Autodesk Inventor part; units mm, degrees
ref_plane "YZ Plane" through (0, 0, 0) normal (1, 0, 0) x (0, 1, 0)
ref_plane "XZ Plane" through (0, 0, 0) normal (0, 1, 0) x (-1, 0, 0)
ref_plane "XY Plane" through (0, 0, 0) normal (0, 0, 1) x (1, 0, 0)
sketch "Sketch1" plane through (0, 0, 0) normal (0, 1, 0) x (-1, 0, 0)
  line L0 (-26, 36) -> (26, 36)
  line L1 (26, 36) -> (26, -36)
  line L2 (26, -36) -> (-26, -36)
  line L3 (-26, -36) -> (-26, 36)
  line L4 (-26, 36) -> (26, -36) construction
  line L5 (26, 36) -> (-26, -36) construction
  point P0 (0, 0)
  dimension "d0" = 72
  dimension "d1" = 52
extrude "Extrusion1" add sketch "Sketch1" along normal blind 1.6
sketch "Sketch2" plane through (0, 1.6, 0) normal (0, 1, 0) x (1, 0, 0)
  line L0 (-12.5, -33) -> (23, -33) construction
  line L1 (23, -33) -> (23, 33) construction
  line L2 (23, 33) -> (-12.5, 33) construction
  line L3 (-12.5, 33) -> (-12.5, -33) construction
  line L4 (-12.5, -33) -> (23, 33) construction
  line L5 (23, -33) -> (-12.5, 33) construction
  line L6 (26, 36) -> (-26, 36) construction
  line L7 (-26, -36) -> (26, -36) construction
  line L8 (26, -36) -> (26, 36) construction
  line L9 (26, 36) -> (-26, 36) construction
  line L10 (-26, 36) -> (-26, -36) construction
  point P0 (0, 0)
  point P1 (5.25, 0)
  dimension "d4" = 66
  dimension "d5" = 35.5
  dimension "d6" = 3
  dimension "d7" = 3
hole "Hole1" at (-12.5, 1.6, 33) at (-12.5, 1.6, -33) at (23, 1.6, -33) at (23, 1.6, 33) direction (0, -1, 0) diameter 3 end through all
sketch "Sketch3" plane through (0, 1.6, 0) normal (0, 1, 0) x (1, 0, 0)
  line L0 (13, -9) -> (25, -9)
  line L1 (25, -9) -> (25, 29)
  line L2 (25, 29) -> (13, 29)
  line L3 (13, 29) -> (13, -9)
  circle A0 centre (23, 33) radius 1.5 construction
  line L4 (26, -36) -> (26, 36) construction
  point P0 (0, 0)
  dimension "d15" = 38
  dimension "d16" = 12
  dimension "d18" = 4
  dimension "d19" = 1
extrude "Extrusion2" add sketch "Sketch3" along normal blind 14
sketch "Sketch4" plane through (0, 1.6, 0) normal (0, 1, 0) x (1, 0, 0)
  line L0 (7, -33) -> (23, -33)
  line L1 (23, -33) -> (23, -11)
  line L2 (23, -11) -> (7, -11)
  line L3 (7, -11) -> (7, -33)
  line L4 (13, -9) -> (13, 29) construction
  line L5 (13, 29) -> (25, 29) construction
  line L6 (25, 29) -> (25, -9) construction
  line L7 (25, -9) -> (13, -9) construction
  circle A0 centre (23, 33) radius 1.5 construction
  circle A1 centre (-12.5, -33) radius 1.5 construction
  circle A2 centre (-12.5, 33) radius 1.5 construction
  circle A3 centre (23, -33) radius 1.5 construction
  line L8 (-26, -36) -> (26, -36) construction
  line L9 (26, -36) -> (26, 36) construction
  line L10 (26, 36) -> (-26, 36) construction
  line L11 (-26, 36) -> (-26, -36) construction
  point P0 (0, 0)
  dimension "d22" = 22
  dimension "d23" = 16
extrude "Extrusion3" add sketch "Sketch4" along normal blind 15
sketch "Sketch5" plane through (0, 1.6, 0) normal (0, 1, 0) x (1, 0, 0)
  line L0 (-25, -28) -> (-6, -28)
  line L1 (-6, -28) -> (-6, 27)
  line L2 (-6, 27) -> (-25, 27)
  line L3 (-25, 27) -> (-25, -28)
  line L4 (-26, -36) -> (26, -36)
  line L5 (-26, 36) -> (-26, -36)
  point P0 (0, 0)
  dimension "d26" = 55
  dimension "d27" = 19
  dimension "d28" = 8
  dimension "d29" = 1
extrude "Extrusion4" add sketch "Sketch5" along normal blind 16
sketch "Sketch6" plane through (0, 0, 0) normal (0, -1, 0) x (1, 0, 0)
  circle A0 centre (23, 33) radius 1.5
  circle A1 centre (23, -33) radius 1.5
  circle A2 centre (-12.5, -33) radius 1.5
  circle A3 centre (-12.5, 33) radius 1.5
  line L0 (25.75, 31.4123) -> (23, 29.8246)
  line L1 (23, 29.8246) -> (20.25, 31.4123)
  line L2 (20.25, 31.4123) -> (20.25, 34.5877)
  line L3 (20.25, 34.5877) -> (23, 36.1754)
  line L4 (23, 36.1754) -> (25.75, 34.5877)
  line L5 (25.75, 34.5877) -> (25.75, 31.4123)
  line L6 (20.25, -31.4123) -> (23, -29.8246)
  line L7 (23, -29.8246) -> (25.75, -31.4123)
  line L8 (25.75, -31.4123) -> (25.75, -34.5877)
  line L9 (25.75, -34.5877) -> (23, -36.1754)
  line L10 (23, -36.1754) -> (20.25, -34.5877)
  line L11 (20.25, -34.5877) -> (20.25, -31.4123)
  line L12 (-9.75, 31.4123) -> (-12.5, 29.8246)
  line L13 (-12.5, 29.8246) -> (-15.25, 31.4123)
  line L14 (-15.25, 31.4123) -> (-15.25, 34.5877)
  line L15 (-15.25, 34.5877) -> (-12.5, 36.1754)
  line L16 (-12.5, 36.1754) -> (-9.75, 34.5877)
  line L17 (-9.75, 34.5877) -> (-9.75, 31.4123)
  line L18 (-9.75, -31.4123) -> (-9.75, -34.5877)
  line L19 (-9.75, -34.5877) -> (-12.5, -36.1754)
  line L20 (-12.5, -36.1754) -> (-15.25, -34.5877)
  line L21 (-15.25, -34.5877) -> (-15.25, -31.4123)
  line L22 (-15.25, -31.4123) -> (-12.5, -29.8246)
  line L23 (-12.5, -29.8246) -> (-9.75, -31.4123)
  line L24 (26, -36) -> (26, 36)
  line L25 (-26, 36) -> (-26, -36)
  point P0 (0, 0)
  dimension "d32" = 5.5
  dimension "d33" = 5.5
  dimension "d34" = 5.5
  dimension "d35" = 5.5
extrude "Extrusion5" add sketch "Sketch6" along normal blind 5
properties part number "backboard"
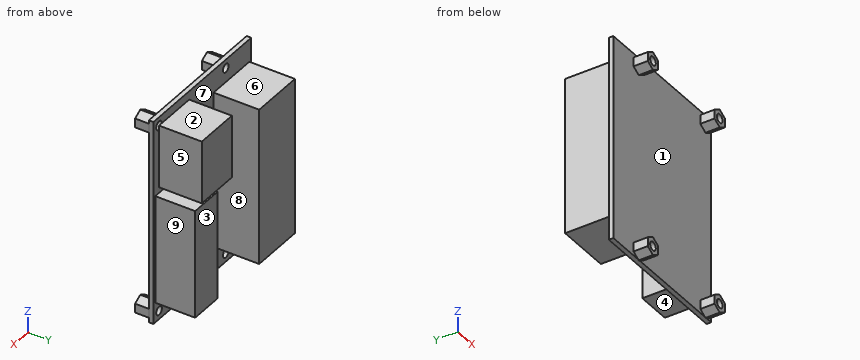
Work out the finished part from the listing and answer in its coordinate system (mm). Face numbers are marked on the shaded views. A direction names the side the tool comes from. Coordinates: 2 decimals unless noted, no trailing zeros. Write each loop counter-clockwise with the first axis right and the second up, starting at its lowest first coordinate (ties: lowest second). Pieces come first, ordered by that corner, then holes.
1. Flat-ended cylindrical pins translate along their axes: pin 1 (10 mm diameter, centred on x = -7, y = 1.5, fed in from -Z); pin 2 (3.5 mm diameter, centred on x = 22, y = 9.5, fed in from +Z); pin 3 (3 mm diameter, centred on x = -5.5, y = 7, fed in from +Z). Find the tip coordinate at first contact, or state that the pin passes through.
Results list:
pin 1: stops at z = -36
pin 2: stops at z = 33
pin 3: stops at z = 28
2. For the marked faces 1, 2, 3, 4 and 5, determine the directions among +Z, -Z, +X, -X, +Y, -Y from which every point of the face is accessible in a straight line to the end or side of a thin tool.
Results list:
face 1: -Y
face 2: +Z, +X, -X, +Y
face 3: -Z, +X, +Y
face 4: -Z, +X, -X, +Y
face 5: +Z, +X, +Y
3. The part is cut by section C-C, the plane x = -8. Write down the section's boundary in (y, z).
Results list:
outline: (0, -36) - (1.6, -36) - (1.6, -27) - (17.6, -27) - (17.6, 28) - (1.6, 28) - (1.6, 36) - (0, 36) - close
4. For a pull along X with two mould halves and no side action, classify the marked faces 6, 7, 8 and 9 as +X half, -X half, draft (parallel to the pull), parting line (faces both ways), or undercut.
Results list:
face 6: draft
face 7: undercut
face 8: undercut
face 9: +X half
5. The part is cut by section A-A, the plane y = 6. Write down the section's boundary in (x, z).
Results list:
outline: (-25, -27) - (-6, -27) - (-6, 28) - (-25, 28) - close; (7, 11) - (23, 11) - (23, 33) - (7, 33) - close; (13, -29) - (25, -29) - (25, 9) - (13, 9) - close
6. Consider line 1 along X through (y, z) = (-3.95, 33); line 2 along X through (y, z) = (0.45, -33); line 3 along Z through (x, y) = (-12.5, 0.3). Determine where each line is inside the solid, lowest interval first.
Results list:
line 1: x = -15.25 to -14, -11 to -9.75, 20.25 to 21.5, 24.5 to 25.75
line 2: x = -26 to -14, -11 to 21.5, 24.5 to 26
line 3: z = -36 to -34.5, -31.5 to 31.5, 34.5 to 36
7. The part is cut by section B-B, the plane z = -33. Write down the section's boundary in (x, y), and give its area (3 significant figures).
Results list:
outline: (-26, 0) - (-15.25, 0) - (-15.25, -5) - (-14, -5) - (-14, 1.6) - (-26, 1.6) - close; (-11, -5) - (-9.75, -5) - (-9.75, 0) - (20.25, 0) - (20.25, -5) - (21.5, -5) - (21.5, 1.6) - (-11, 1.6) - close; (24.5, -5) - (25.75, -5) - (25.75, 0) - (26, 0) - (26, 1.6) - (24.5, 1.6) - close
area: 98.6 mm2
8. The part is cut by section D-D, the plane z = 23. Write down the section's boundary in (x, y), and give its area (3 significant figures).
Results list:
outline: (-26, 0) - (26, 0) - (26, 1.6) - (23, 1.6) - (23, 16.6) - (7, 16.6) - (7, 1.6) - (-6, 1.6) - (-6, 17.6) - (-25, 17.6) - (-25, 1.6) - (-26, 1.6) - close
area: 627 mm2
